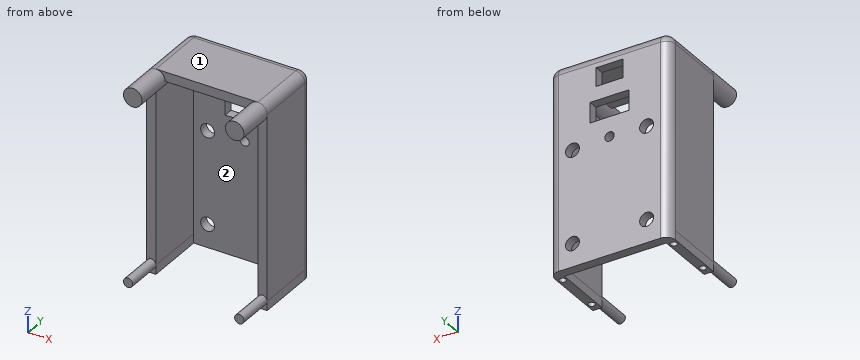
from build123d import *

# Parameters (mm, degrees)
SKETCH1_W                       = 33.02
SKETCH1_H                       = 55.88
BOSS_EXTRUDE1_DEPTH             = 19.05
SHELL2_T                        = -2.54
FILLET2_R                       = 2.54
SKETCH2_R                       = 1.905
CUT_EXTRUDE1_DEPTH              = 2.54
CUT_EXTRUDE2_REACH              = 69.645
SKETCH3_W                       = 10.668
SKETCH3_H                       = 5.588
CUT_EXTRUDE3_REACH              = 69.645
SKETCH4_R                       = 1.27
CUT_EXTRUDE4_REACH              = 69.645
SKETCH5_W                       = 7.366
SKETCH5_H                       = 5.08
BOSS_EXTRUDE2_START             = -16.51
SKETCH6_R                       = 2.54
SKETCH6_R_2                     = 1.27
BOSS_EXTRUDE2_DEPTH             = 26.67
F_49_0_073_DIAMETER_HOLE1_D     = 1.8542
F_49_0_073_DIAMETER_HOLE1_DEPTH = 8.89
F_49_0_073_DIAMETER_HOLE1_TIP   = 0.55705788


with BuildPart() as part:
    # Sketch1 → Boss-Extrude1 (new body)
    with BuildSketch(Plane(origin=(0, 0, 0), x_dir=(1, 0, 0), z_dir=(0, 1, 0))):
        with Locations((16.51, 27.94)):
            Rectangle(SKETCH1_W, SKETCH1_H)
    extrude(amount=BOSS_EXTRUDE1_DEPTH)

    # Shell2
    shell2_openings = [part.faces().sort_by_distance(p)[0] for p in [
        (16.51, 0, -27.94),
        (16.51, 9.525, -55.88),
    ]]
    offset(amount=SHELL2_T, openings=shell2_openings, kind=Kind.INTERSECTION)

    # Fillet2
    fillet2_edges = [part.edges().sort_by_distance(p)[0] for p in [
        (33.02, 19.05, -27.94),
        (0, 19.05, -27.94),
        (16.51, 19.05, 0),
        (33.02, 9.525, 0),
        (0, 9.525, 0),
    ]]
    fillet(fillet2_edges, radius=FILLET2_R)

    # Sketch2 → Cut-Extrude1 (cut)
    with BuildSketch(Plane(origin=(0, 19.05, 0), x_dir=(1, 0, 0), z_dir=(0, 1, 0))):
        with Locations(Location((26.67, 49.53, 0), (0, 0, 270))):
            Circle(SKETCH2_R)
        with Locations(Location((26.67, 24.13, 0), (0, 0, 270))):
            Circle(SKETCH2_R)
        with Locations(Location((6.35, 24.13, 0), (0, 0, 270))):
            Circle(SKETCH2_R)
        with Locations(Location((6.35, 49.53, 0), (0, 0, 270))):
            Circle(SKETCH2_R)
    extrude(amount=-CUT_EXTRUDE1_DEPTH, mode=Mode.SUBTRACT)

    # Sketch3 → Cut-Extrude2 (cut, up to next)
    with BuildSketch(Plane(origin=(0, 19.05, 0), x_dir=(1, 0, 0), z_dir=(0, 1, 0)), mode=Mode.PRIVATE) as cut_extrude2_sk1:
        with Locations((16.51, 15.494)):
            Rectangle(SKETCH3_W, SKETCH3_H)
    cut_extrude2_tool1 = extrude(cut_extrude2_sk1.sketch, amount=-CUT_EXTRUDE2_REACH, mode=Mode.PRIVATE) & part.part
    add(cut_extrude2_tool1.solids().sort_by_distance((16.51, 19.05, -15.494))[0], mode=Mode.SUBTRACT)

    # Sketch4 → Cut-Extrude3 (cut, up to next)
    with BuildSketch(Plane(origin=(0, 19.05, 0), x_dir=(1, 0, 0), z_dir=(0, 1, 0)), mode=Mode.PRIVATE) as cut_extrude3_sk1:
        with Locations(Location((16.51, 23.687982585, 0), (0, 0, 270))):
            Circle(SKETCH4_R)
    cut_extrude3_tool1 = extrude(cut_extrude3_sk1.sketch, amount=-CUT_EXTRUDE3_REACH, mode=Mode.PRIVATE) & part.part
    add(cut_extrude3_tool1.solids().sort_by_distance((16.51, 19.05, -23.687983))[0], mode=Mode.SUBTRACT)

    # Sketch5 → Cut-Extrude4 (cut, up to next)
    with BuildSketch(Plane(origin=(0, 19.05, 0), x_dir=(1, 0, 0), z_dir=(0, 1, 0)), mode=Mode.PRIVATE) as cut_extrude4_sk1:
        with Locations((16.51, 6.35)):
            Rectangle(SKETCH5_W, SKETCH5_H)
    cut_extrude4_tool1 = extrude(cut_extrude4_sk1.sketch, amount=-CUT_EXTRUDE4_REACH, mode=Mode.PRIVATE) & part.part
    add(cut_extrude4_tool1.solids().sort_by_distance((16.51, 19.05, -6.35))[0], mode=Mode.SUBTRACT)

    # Sketch6 → Boss-Extrude2 (add)
    with BuildSketch(Plane(origin=(0, 0, 0), x_dir=(-1, 0, 0), z_dir=(0, -1, 0)).offset(BOSS_EXTRUDE2_START)):
        with Locations(Location((-30.48, 2.54, 0), (0, 0, 90))):
            Circle(SKETCH6_R)
        with Locations(Location((-2.54, 2.54, 0), (0, 0, 90))):
            Circle(SKETCH6_R)
        with Locations(Location((-31.75, 53.34, 0), (0, 0, 90))):
            Circle(SKETCH6_R_2)
        with Locations(Location((-1.27, 53.34, 0), (0, 0, 90))):
            Circle(SKETCH6_R_2)
    extrude(amount=BOSS_EXTRUDE2_DEPTH)

    # #49 (0.073) Diameter Hole1
    with Locations(Plane(origin=(0, 0, -55.88), x_dir=(-1, 0, 0), z_dir=(0, 0, -1))):
        with Locations((-31.75, 15.24), (-31.75, 2.54), (-1.27, 2.54), (-1.27, 15.24)):
            Hole(F_49_0_073_DIAMETER_HOLE1_D / 2, depth=F_49_0_073_DIAMETER_HOLE1_DEPTH)
            with Locations((0, 0, -(F_49_0_073_DIAMETER_HOLE1_DEPTH + F_49_0_073_DIAMETER_HOLE1_TIP / 2))):  # 118° drill point
                Cone(0, F_49_0_073_DIAMETER_HOLE1_D / 2, F_49_0_073_DIAMETER_HOLE1_TIP, mode=Mode.SUBTRACT)


solid = part.part
Source: CAD feature listing. Evaluate the final solid. Frame: model axes, mm. Face numbers are marked on the shaded views. Give positions to 0.01 mm unless a question says otherwise; leave off trailing zeros. Write each loop counter-clockwise with the first axis right and the second up, starting at its lowest first coordinate (ties: lowest second). Pieces come first, ordered by that corner, then holes. Notation, with made-up numbers: (-36.5, 0.5) -> (-23.5, 0.5) arc R26 cw to (-23.5, 18.5) -> close; hole circle Ø5 at (-2, 40). An arc over 180 degrees is marked (long way). Return JSON: item names as keys, results as strings. Group by question number.
1. Mould query, pull axis X, two halves, no side actions, for the marked faces 1 and 2. Classes: +X half, -X half, draft (parallel to the pull), parting line (faces both ways), or undercut.
2. Section D-D, the plane z = -24.13. Output: boundary loops of the cut face in (x, y) (3 decimals).
3. Material intervals for line 1 (X direction, y = 3, z = -43); line 2 (X direction, y = 18.45, z = -49.53) (3 decimals); line 3 (X direction, y = 3, z = -52.5), sorted ascending. Write a range as from..to.
4. Pin query (flat end, axial travel): pin 1 Ø3.5 at (x, z) = (6.35, -49.53) entering from -Y; pin 2 Ø5 at (x, y) = (21, 9.5) entering from -Z; pin 3 Ø2 at (y, z) = (18, -5) entering from -X; pin 4 Ø6 at (x, z) = (26.67, -24.13) entering from -Y. Return the tip coordinate at first contact, or that it passes through.
5. Section C-C, the plane z = -7.5. Output: boundary loops of the cut face in (x, y).
6. Section B-B, the plane x = 26.67. Output: boundary loops of the cut face in (y, z) (3 decimals), then the cut area to 3 significant figures.
7. Section A-A, the plane z = -49.53. Output: boundary loops of the cut face in (x, y) (3 decimals), then the cut area to 3 significant figures.
Determined:
{
 "1": {"face 1": "draft", "face 2": "undercut"},
 "2": {"outline": "(0, 0) -> (2.54, 0) -> (2.54, 16.51) -> (4.445, 16.51) -> (4.445, 19.05) -> (2.54, 19.05) arc R2.54 ccw to (0, 16.51) -> close; (8.255, 16.51) -> (15.319, 16.51) -> (15.319, 19.05) -> (8.255, 19.05) -> close; (17.701, 16.51) -> (24.765, 16.51) -> (24.765, 19.05) -> (17.701, 19.05) -> close; (28.575, 16.51) -> (30.48, 16.51) -> (30.48, 0) -> (33.02, 0) -> (33.02, 16.51) arc R2.54 ccw to (30.48, 19.05) -> (28.575, 19.05) -> close"},
 "3": {"line 1": "x = 0..2.54, 30.48..33.02", "line 2": "x = 0.9..4.445, 8.255..24.765, 28.575..32.12", "line 3": "x = 0..0.47, 2.07..2.54, 30.48..30.95, 32.55..33.02"},
 "4": {"pin 1": "passes through", "pin 2": "stops at z = -2.54", "pin 3": "stops at x = 0.05", "pin 4": "stops at y = 16.51"},
 "5": {"outline": "(0, 0) -> (2.54, 0) -> (2.54, 16.51) -> (12.83, 16.51) -> (12.83, 19.05) -> (2.54, 19.05) arc R2.54 ccw to (0, 16.51) -> close; (20.19, 16.51) -> (30.48, 16.51) -> (30.48, 0) -> (33.02, 0) -> (33.02, 16.51) arc R2.54 ccw to (30.48, 19.05) -> (20.19, 19.05) -> close"},
 "6": {"outline": "(0, -2.54) -> (16.51, -2.54) -> (16.51, -22.225) -> (19.05, -22.225) -> (19.05, -2.54) arc R2.54 ccw to (16.51, 0) -> (0, 0) -> close; (16.51, -55.88) -> (19.05, -55.88) -> (19.05, -51.435) -> (16.51, -51.435) -> close; (16.51, -47.625) -> (19.05, -47.625) -> (19.05, -26.035) -> (16.51, -26.035) -> close", "area": "163 mm2"},
 "7": {"outline": "(0, 0) -> (2.54, 0) -> (2.54, 16.51) -> (4.445, 16.51) -> (4.445, 19.05) -> (2.54, 19.05) arc R2.54 ccw to (0, 16.51) -> close; (8.255, 16.51) -> (24.765, 16.51) -> (24.765, 19.05) -> (8.255, 19.05) -> close; (28.575, 16.51) -> (30.48, 16.51) -> (30.48, 0) -> (33.02, 0) -> (33.02, 16.51) arc R2.54 ccw to (30.48, 19.05) -> (28.575, 19.05) -> close; hole circle Ø1.854 at (1.27, 2.54); hole circle Ø1.854 at (1.27, 15.24); hole circle Ø1.854 at (31.75, 2.54); hole circle Ø1.854 at (31.75, 15.24)", "area": "135 mm2"}
}
